For this review, take the finished solid that the model builds, in its own axes (mm). A direction names the side the tool comes from. Coordinates: 2 decimals unless noted, no trailing zeros. Loops run counter-clockwise (first coordinate to the right, second up) from the corner with the lowest first, then second, coordinate; pieces in that order, holes last. Notation, with made-up numbers: M -33,-26 L 21,-26 A20 ccw 21,-15 Z; hole C 60,43.25 d4. An arc over 180 degrees is marked long. Answer as a JSON object with one key per item and string values. Group by question number.
Item 1: Add section D-D (z = 8). State the section outline as (x, y) points.
Item 2: Add section A-A (x = 0). State the section outline as (y, z) points.
Item 3: Mouldability with a two-part tool opening along Z and no side actions: class faces 5 (the face through (14.71, -0.04, -8.52)), 6 (the face through (11.6, -2.11, 3.11)), 7 (the face through (16.746, -0.042, 2.926)) as +Z half, -Z half, draft (parallel to the pull), parting line (faces both ways), or undercut.
Item 4: Wall thickness on L1, parallel to Z at x = 0, y = -0.5; L2, parallel to Y at x = -5.5, z = -12; L3, parallel to Z at x = 0, y = -2.25: over which ranges is each line inside the solid? List them lowest first. Write a range as from..to.
Item 5: Add section C-C (z = 0). State the section outline as (x, y) points, then the cut area to 3 significant figures.
Item 6: Insertion check: pin 1 (3 mm diameter, centred on x = 11, z = -1.5, fed in from +Y); pin 2 (1.8 mm diameter, centred on x = -10, z = 2.5, fed in from -Y); pin 3 (1.5 mm diameter, centred on x = 11, y = -0.5, fed in from -Z). Each pin has a flat end and moves straight along its axis. Give the tip position at first contact, or say it passes through.
Item 7: Tool access review of faces 1 (the face through (9.4, -3.5, -12.2)), 2 (the face through (13.453, 0.042, 7.7)), 3 (the face through (-11.6, -0.36, 3.11)), 4 (the face through (3.518, -1.663, 9.468)): name each direction out of +Z, -Z, +X, -X, +Y, -Y from which nothing blocks a thin tool from reaching the whole face with its end or side.
Item 8: Add section B-B (y = 1.75). State the section outline as (x, z) points, then the cut area to 3 significant figures.
from build123d import *
from build123d.topology import SkipClean

# Parameters (mm, degrees)
EXTRUDE_1_DEPTH                  = 3
SKETCH_3_R                       = 15.4
EXTRUDE_2_DEPTH                  = 1
SKETCH_4_R                       = 13.4
CUT_EXTRUDE_1_DEPTH              = 68.538877693
EXTRUDE_3_DEPTH                  = 3.5
CUT_EXTRUDE_START                = -1.7
CUT_EXTRUDE_2_DEPTH              = 1.7
FILLET_1_R                       = 0.5
PATTERN_CIRCULAR_1_COUNT         = 4
FILLET_1_OF_PATTERN_CIRCULAR_1_R = 0.5
HOLE_WIZARD_M2_1_D               = 2.4
HOLE_WIZARD_M2_1_CBORE_D         = 5
HOLE_WIZARD_M2_1_CBORE_DEPTH     = 1.6
HOLE_WIZARD_M2_2_D               = 2.4
HOLE_WIZARD_M2_2_CBORE_D         = 5
HOLE_WIZARD_M2_2_CBORE_DEPTH     = 1.6
HOLE_WIZARD_M2_1_2_D             = 1.6
FILLET_2_R                       = 3
CUT_EXTRUDE_START_2              = -1.6
SKETCH_15_R                      = 2.5
CUT_EXTRUDE_4_DEPTH              = 1.6
SKETCH_16_W                      = 105
SKETCH_16_H                      = 105
SKETCH_16_R                      = 17
CUT_EXTRUDE_5_DEPTH              = 68.44256816
SKETCH_17_R                      = 8.333697596
CUT_EXTRUDE_6_DEPTH              = 10
PATTERN_CIRCULAR_2_COUNT         = 9


with BuildPart() as part:
    # ｽｹｯﾁ2 → ﾎﾞｽ - 押し出し1 (new, symmetric)
    with BuildSketch(Plane(origin=(0, 0, 0), x_dir=(1, 0, 0), z_dir=(0, 1, 0))):
        with BuildLine():
            ThreePointArc((-13.5, 23.382685902), (-18.457166085, 19.706167058), (-22.449944321, 15))
            Line((-22.449944321, 15), (-13.5, 15))
            Line((-13.5, 15), (-13.5, 23.382685902))
        make_face()
        with BuildLine():
            Line((13.5, 15), (22.449944321, 15))
            ThreePointArc((22.449944321, 15), (18.457166085, 19.706167058), (13.5, 23.382685902))
            Line((13.5, 23.382685902), (13.5, 15))
        make_face()
        with BuildLine():
            Line((-47.5, 0), (-27, 0))
            ThreePointArc((-27, 0), (0, -27), (27, 0))
            Line((27, 0), (47.5, 0))
            Line((47.5, 0), (47.5, 15))
            Line((47.5, 15), (22.449944321, 15))
            Line((22.449944321, 15), (13.5, 15))
            Line((13.5, 15), (13.5, 23.382685902))
            ThreePointArc((13.5, 23.382685902), (0, 27), (-13.5, 23.382685902))
            Line((-13.5, 23.382685902), (-13.5, 15))
            Line((-13.5, 15), (-22.449944321, 15))
            Line((-22.449944321, 15), (-47.5, 15))
            Line((-47.5, 15), (-47.5, 0))
        make_face()
        with BuildLine():
            Line((-13.5, 47.5), (-13.5, 23.382685902))
            ThreePointArc((-13.5, 23.382685902), (0, 27), (13.5, 23.382685902))
            Line((13.5, 23.382685902), (13.5, 47.5))
            Line((13.5, 47.5), (-13.5, 47.5))
        make_face()
    extrude(amount=EXTRUDE_1_DEPTH, both=True)

    # ｽｹｯﾁ3 → ﾎﾞｽ - 押し出し2 (add)
    with BuildSketch(Plane.XZ.offset(3)):
        with Locations(Location((0, 0, 0), (0, 0, 90))):
            Circle(SKETCH_3_R)
    extrude(amount=EXTRUDE_2_DEPTH)

    # ｽｹｯﾁ4 → ｶｯﾄ - 押し出し1 (cut, through all)
    with BuildSketch(Plane.XZ.offset(4)):
        with Locations(Location((0, 0, 0), (0, 0, 270))):
            Circle(SKETCH_4_R)
    extrude(amount=-CUT_EXTRUDE_1_DEPTH, mode=Mode.SUBTRACT)

    # ｽｹｯﾁ5 → ﾎﾞｽ - 押し出し3 (add)
    with BuildSketch(Plane.XZ.offset(3)):
        with BuildLine():
            Line((-7.079183569, -7.203829536), (-9.392184142, -9.557556019))
            ThreePointArc((-9.392184142, -9.557556019), (-3.411666106, -12.958415581), (3.468175204, -12.943406072))
            Line((3.468175204, -12.943406072), (2.614072356, -9.755850846))
            ThreePointArc((2.614072356, -9.755850846), (-2.571479677, -9.767163983), (-7.079183569, -7.203829536))
        make_face()
    extrude_3 = extrude(amount=-EXTRUDE_3_DEPTH)

    # ｽｹｯﾁ6 → ｶｯﾄ - 押し出し2 (cut)
    with SkipClean():  # the faces are left unmerged after this step: merging them gives an invalid solid
        with BuildSketch(Plane(origin=(0, 0.5, 0), x_dir=(1, 0, 0), z_dir=(0, 1, 0)).offset(CUT_EXTRUDE_START)):
            with BuildLine():
                Line((-3.468175204, 12.943406072), (0, 0))
                Line((0, 0), (3.468175204, 12.943406072))
                ThreePointArc((3.468175204, 12.943406072), (0, 13.4), (-3.468175204, 12.943406072))
            make_face()
        cut_extrude_2 = extrude(amount=CUT_EXTRUDE_2_DEPTH, mode=Mode.SUBTRACT)

    # ﾌｨﾚｯﾄ1
    fillet_1_edges = [part.edges().sort_by_distance(p)[0] for p in [
        (-7.079183569, -1.25, -7.203829536),
        (2.614072356, -2.1, -9.755850846),
        (-2.614072356, -0.35, -9.755850846),
    ]]
    fillet(fillet_1_edges, radius=FILLET_1_R)

    # 円形ﾊﾟﾀｰﾝ1: ﾎﾞｽ - 押し出し3, ｶｯﾄ - 押し出し2 ×4 about axis
    with SkipClean():  # the faces are left unmerged after this step: merging them gives an invalid solid
        pattern_circular_1_axis = Axis((0, 0, 0), (0, 1, 0))
        add([extrude_3.rotate(pattern_circular_1_axis, i * 360 / PATTERN_CIRCULAR_1_COUNT) for i in range(1, PATTERN_CIRCULAR_1_COUNT)])
        add([cut_extrude_2.rotate(pattern_circular_1_axis, i * 360 / PATTERN_CIRCULAR_1_COUNT) for i in range(1, PATTERN_CIRCULAR_1_COUNT)], mode=Mode.SUBTRACT)

    # ﾌｨﾚｯﾄ1 of 円形ﾊﾟﾀｰﾝ1
    fillet_1_of_pattern_circular_1_edges = [part.edges().sort_by_distance(p)[0] for p in [
        (-7.203829536, -1.25, 7.079183569),
        (-9.755850846, -2.1, -2.614072356),
        (-9.755850846, -0.35, 2.614072356),
        (7.079183569, -1.25, 7.203829536),
        (-2.614072356, -2.1, 9.755850846),
        (2.614072356, -0.35, 9.755850846),
        (7.203829536, -1.25, -7.079183569),
        (9.755850846, -2.1, 2.614072356),
        (9.755850846, -0.35, -2.614072356),
    ]]
    fillet(fillet_1_of_pattern_circular_1_edges, radius=FILLET_1_OF_PATTERN_CIRCULAR_1_R)

    # Hole Wizard M2 _1 (through all)
    with Locations(Plane(origin=(0, 3, 0), x_dir=(1, 0, 0), z_dir=(0, 1, 0))):
        with Locations((-10.5, -22.5), (-22.5, -10.5)):
            hole_wizard_m2_1 = CounterBoreHole(HOLE_WIZARD_M2_1_D / 2, HOLE_WIZARD_M2_1_CBORE_D / 2, HOLE_WIZARD_M2_1_CBORE_DEPTH)

    # M2 なべ頭ねじ用座ぐり穴2 (through all)
    with Locations(Plane(origin=(0, -3, 0), x_dir=(-1, 0, 0), z_dir=(0, -1, 0))):
        with Locations((10.5, 21), (10.5, 42), (22.5, 10.5)):
            hole_wizard_m2_2 = CounterBoreHole(HOLE_WIZARD_M2_2_D / 2, HOLE_WIZARD_M2_2_CBORE_D / 2, HOLE_WIZARD_M2_2_CBORE_DEPTH)

    # Hole Wizard M2 _1 2 (through all)
    with Locations(Plane(origin=(0, -3, 0), x_dir=(-1, 0, 0), z_dir=(0, -1, 0))):
        with Locations((43.5, 12), (10.5, 43.5)):
            hole_wizard_m2_1_2 = Hole(HOLE_WIZARD_M2_1_2_D / 2)

    # ﾐﾗｰ1: Hole Wizard M2 _1, M2 なべ頭ねじ用座ぐり穴2, Hole Wizard M2 _1 2 across plane
    with SkipClean():  # the faces are left unmerged after this step: merging them gives an invalid solid
        add(hole_wizard_m2_1.mirror(Plane(origin=(0, 0, 0), x_dir=(0, 0, 1), z_dir=(1, 0, 0))), mode=Mode.SUBTRACT)
        add(hole_wizard_m2_2.mirror(Plane(origin=(0, 0, 0), x_dir=(0, 0, 1), z_dir=(1, 0, 0))), mode=Mode.SUBTRACT)
        add(hole_wizard_m2_1_2.mirror(Plane(origin=(0, 0, 0), x_dir=(0, 0, 1), z_dir=(1, 0, 0))), mode=Mode.SUBTRACT)

    # ﾌｨﾚｯﾄ2
    fillet_2_edges = [part.edges().sort_by_distance(p)[0] for p in [
        (47.5, 0, -15),
        (47.5, 0, 0),
        (27, 0, 0),
        (-27, 0, 0),
        (-47.5, 0, 0),
        (-47.5, 0, -15),
        (-22.449944321, 0, -15),
        (-13.5, 0, -23.382685902),
        (-13.5, 0, -47.5),
        (13.5, 0, -47.5),
        (13.5, 0, -23.382685902),
        (22.449944321, 0, -15),
    ]]
    fillet(fillet_2_edges, radius=FILLET_2_R)

    # ｽｹｯﾁ15 → ｶｯﾄ - 押し出し4 (cut)
    with SkipClean():  # the faces are left unmerged after this step: merging them gives an invalid solid
        with BuildSketch(Plane.XZ.offset(3).offset(CUT_EXTRUDE_START_2)):
            with Locations((-22.5, 10.5)):
                Circle(SKETCH_15_R)
            with Locations((22.5, 10.5)):
                Circle(SKETCH_15_R)
        extrude(amount=CUT_EXTRUDE_4_DEPTH, mode=Mode.SUBTRACT)

    # ｽｹｯﾁ16 → ｶｯﾄ - 押し出し5 (cut, through all)
    with SkipClean():  # the faces are left unmerged after this step: merging them gives an invalid solid
        with BuildSketch(Plane.XZ.offset(3)):
            Rectangle(SKETCH_16_W, SKETCH_16_H)
            with Locations(Location((0, 0, 0), (0, 0, 270))):
                Circle(SKETCH_16_R, mode=Mode.SUBTRACT)
        extrude(amount=-CUT_EXTRUDE_5_DEPTH, mode=Mode.SUBTRACT)

    # ｽｹｯﾁ17 → ｶｯﾄ - 押し出し6 (cut)
    with SkipClean():  # the faces are left unmerged after this step: merging them gives an invalid solid
        with BuildSketch(Plane(origin=(0, 3, 0), x_dir=(1, 0, 0), z_dir=(0, 1, 0))):
            with Locations((0, 23.833697596)):
                Circle(SKETCH_17_R)
        cut_extrude_6 = extrude(amount=-CUT_EXTRUDE_6_DEPTH, mode=Mode.SUBTRACT)

    # 円形ﾊﾟﾀｰﾝ2: ｶｯﾄ - 押し出し6 ×9 about axis
    with SkipClean():  # the faces are left unmerged after this step: merging them gives an invalid solid
        pattern_circular_2_axis = Axis((0, 0, 0), (0, 1, 0))
        for i in range(1, PATTERN_CIRCULAR_2_COUNT):
            add(cut_extrude_6.rotate(pattern_circular_2_axis, i * 360 / PATTERN_CIRCULAR_2_COUNT), mode=Mode.SUBTRACT)


solid = part.part
From the geometry:
{
 "1": {"outline": "M -13.28,-3 L -13.16,-3 L -13.16,-4 L -10.75,-4 L -10.75,-3 L -8.14,-3 L -8.14,0.5 L -10.75,0.5 L -10.75,3 L -13.28,3 Z; M 6.17,-3 L 7.86,-3 L 7.86,0.5 L 6.17,0.5 Z; M 10.75,-4 L 13.16,-4 L 13.16,-3 L 13.28,-3 L 13.28,3 L 10.75,3 Z"},
 "2": {"outline": "M -4,-15.4 L -3,-15.4 L -3,-15.5 L 3,-15.5 L 3,-13.4 L -1.2,-13.4 L -1.2,-10.1 L -3,-10.1 L -3,-13.4 L -4,-13.4 Z; M -4,13.4 L -3,13.4 L -3,10.1 L -1.2,10.1 L -1.2,13.4 L 3,13.4 L 3,17 L -3,17 L -3,15.4 L -4,15.4 Z"},
 "3": {"face 5": "-Z half", "face 6": "undercut", "face 7": "+Z half"},
 "4": {"L1": "z = -15.5..-13.4, 13.4..17", "L2": "y = -3..0.5", "L3": "z = -15.5..-10.1, 10.1..17"},
 "5": {"outline": "M -16.24,-3 L -15.4,-3 L -15.4,-4 L -13.4,-4 L -13.4,-3 L -10.1,-3 L -10.1,-1.2 L -13.4,-1.2 L -13.4,3 L -16.24,3 Z; M 10.1,-3 L 13.4,-3 L 13.4,-4 L 15.4,-4 L 15.4,-3 L 16.24,-3 L 16.24,3 L 13.4,3 L 13.4,-1.2 L 10.1,-1.2 Z", "area": "49.9 mm²"},
 "6": {"pin 1": "stops at y = 0.5", "pin 2": "stops at y = -3", "pin 3": "stops at z = -11.64"},
 "7": {"face 1": "-Y", "face 2": "+Z, +X, +Y, -Y", "face 3": "+Y", "face 4": "+Y, -Y"},
 "8": {"outline": "M -16.97,1.07 A8.33 cw -15.58,-6.81 A17 ccw -13.68,-10.09 A8.33 cw -7.56,-15.23 A17 ccw -4,-16.52 A8.33 cw 4,-16.52 A17 ccw 7.56,-15.23 A8.33 cw 13.68,-10.09 A17 ccw 15.58,-6.81 A8.33 cw 16.97,1.07 A17 ccw 16.31,4.8 A8.33 cw 12.31,11.73 A17 ccw 9.41,14.16 A8.33 cw 1.89,16.89 A17 ccw -1.89,16.89 A8.33 cw -9.41,14.16 A17 ccw -12.31,11.73 A8.33 cw -16.31,4.8 A17 ccw Z; hole C 0,0 d26.8", "area": "271 mm²"}
}
